Check sheet for the drawn part. Datum: minimum x, y, z corner. Units: mm. Coordinates: 2 decimals unless noted, no trailing zeros. Order: outer loops, then holes, each group sorted by start corner. A loop starts at its lowest first (then second) coordinate and runs counter-clockwise, first axis right, second up.
1. Draft check along Y on the marked faces 1 and 2. Enter one of: released by +Y, released by -Y, zero draft, split by the parting line, or undercut.
2. Cross-section at B-B (y = 0.7). Enter the section's corners in (x, z), then the cut area to 3 significant figures.
3. Cross-section at D-D (x = 15). Enter the section's corners in (y, z) (1 decimal).
4. Gauge pin test, flat ends, axial feed: pin 1 Ø4 at (x, z) = (39, 27) entering from -Y; pin 2 Ø2.5 at (x, z) = (27.5, 15) entering from -Y; pin 3 Ø0.5 at (y, z) = (0.5, 4.5) entering from +X; pin 4 Ø0.5 at (y, z) = (0.5, 4.5) entering from -X. Record the tip position at first contact, or that the pin passes through.
5. Cross-section at A-A (x = 27.5). Enter the section's corners in (y, z).
6. Thickness scan on line 1 (X direction, y = 0.45, z = 27.5); line 2 (X direction, y = 0.85, z = 33) (1 decimal); line 3 (X direction, y = 0.4, z = 33.5) (1 decimal). Record the ranges inside material, lowest first.
7. Cross-section at C-C (z = 21.5). Enter the section's corners in (x, y).
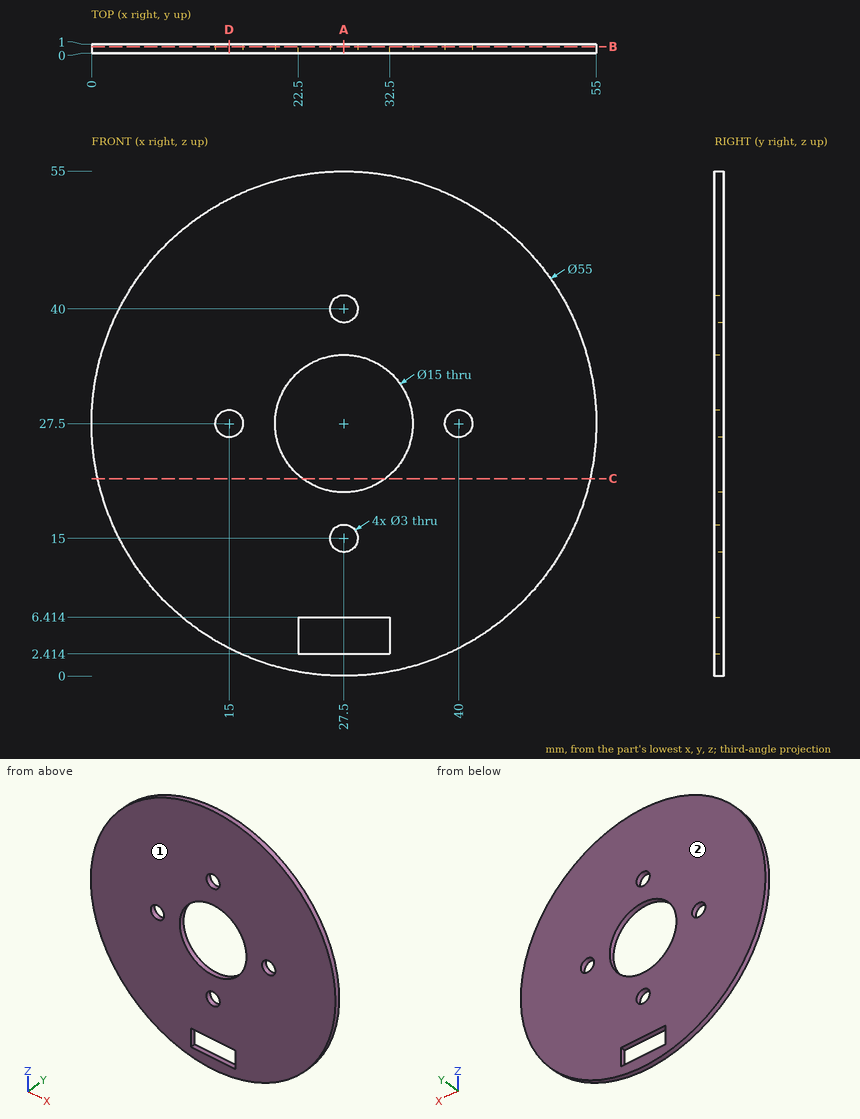
Data:
1. face 1: released by -Y
1. face 2: released by +Y
2. outline: circle Ø55 at (27.5, 27.5); hole circle Ø3 at (15, 27.5); hole circle Ø15 at (27.5, 27.5); hole (22.5, 2.41) - (32.5, 2.41) - (32.5, 6.41) - (22.5, 6.41) - close; hole circle Ø3 at (27.5, 15); hole circle Ø3 at (27.5, 40); hole circle Ø3 at (40, 27.5)
2. area: 2,130 mm2
3. outline: (0, 3) - (1, 3) - (1, 26) - (0, 26) - close; (0, 29) - (1, 29) - (1, 52) - (0, 52) - close
4. pin 1: stops at y = 0
4. pin 2: passes through
4. pin 3: stops at x = 42.95
4. pin 4: stops at x = 12.05
5. outline: (0, 0) - (1, 0) - (1, 2.41) - (0, 2.41) - close; (0, 6.41) - (1, 6.41) - (1, 13.5) - (0, 13.5) - close; (0, 16.5) - (1, 16.5) - (1, 20) - (0, 20) - close; (0, 35) - (1, 35) - (1, 38.5) - (0, 38.5) - close; (0, 41.5) - (1, 41.5) - (1, 55) - (0, 55) - close
6. line 1: x = 0 to 13.5, 16.5 to 20, 35 to 38.5, 41.5 to 55
6. line 2: x = 0.6 to 22.4, 32.6 to 54.4
6. line 3: x = 0.7 to 23, 32 to 54.3
7. outline: (0.66, 0) - (23, 0) - (23, 1) - (0.66, 1) - close; (32, 0) - (54.34, 0) - (54.34, 1) - (32, 1) - close
